The model under review builds one solid part; all positions refer to its coordinate system, in mm. A direction names the side the tool comes from. Give positions to 0.01 mm unless a question says otherwise; leave off trailing zeros. Loops run counter-clockwise (first coordinate to the right, second up) from the corner with the lowest first, then second, coordinate; pieces in that order, holes last. Notation, with made-up numbers: M 67,-4 L 73,-4 A18 cw 73,23 Z; hole C -19,18.25 d1. An arc over 180 degrees is marked long. One line per item, written item: value. Start each with the question number.
Q1. We need section B-B on y = -50.5. Write out the cut boundary in (x, z).
Q2. For pin 1 (3 mm diameter, centred on x = -85.68, y = -111.2, fed in from -Z); pin 2 (3 mm diameter, centred on x = 0, y = -188.04, fed in from +Z); pin 3 (1.5 mm diameter, centred on x = -11, z = 1.5, fed in from -Y); pin 4 (1.5 mm diameter, centred on x = -14, z = 2, fed in from +Y), all flat-tipped, find the tip position at first contact; note any pin that passes through.
Q3. For faces 4 (the face through (-32.17, -58.77, -1.48)), 5 (the face through (1.15, -190.26, 1.52)), list the 3-axis set-ups (+Z, -Z, +X, -X, +Y, -Y) from which the entire face can be reached by the end or side of a thin tool; tool diameter is ignored.
Q4. We need section D-D on y = -158.5. Write out the cut boundary in (x, z).
Q5. We need section C-C on x = -142. Write out the cut boundary in (y, z), plus the area to 3 significant figures.
Q6. We need section A-A on z = -1.2. Write out the cut boundary in (x, y), plus the area to 3 significant figures.
Q7. To check wall thickness, follow line 1 along Y through (x, z) = (0, 2.1); line 2 along X through (y, z) = (-120, 0.2); line 3 along X through (y, z) = (-118, 0.4). State the ranges of each line that lie inside material, in increasing order. Write a range as from..to.
Q8. Mouldability with a two-part tool opening along Y and no side actions: class faces 1 (the face through (-34, -57, -3)), 2 (the face through (-84.53, -149.05, 1.48)), 3 (the face through (-97.158, -125.157, 1.521)) as released by +Y, released by -Y, zero draft, split by the parting line, or undercut.
Autodesk Inventor part; units mm, degrees
ref_plane "YZ Plane" through (0, 0, 0) normal (1, 0, 0) x (0, 1, 0)
ref_plane "XZ Plane" through (0, 0, 0) normal (0, 1, 0) x (-1, 0, 0)
ref_plane "XY Plane" through (0, 0, 0) normal (0, 0, 1) x (1, 0, 0)
sketch "Sketch1" plane through (0, 0, 0) normal (0, 0, 1) x (1, 0, 0)
  line L0 (-169.4076, 105.3841) -> (50.098, -274.8108)
  circle A0 centre (-54.282, -94.0192) radius 2.75
  circle A1 centre (0, 0) radius 8.5
  circle A2 centre (-162.8461, -94.0192) radius 8.5
  circle A3 centre (0, -188.0385) radius 8.5
  line L1 (0, 0) -> (0, -188.0385)
  line L2 (0, -188.0385) -> (-162.8461, -94.0192)
  line L3 (-162.8461, -94.0192) -> (0, 0)
  line L4 (38.7758, 32.2022) -> (-208.87, -110.7762)
  line L5 (8.5, -269.7975) -> (8.5, 26.6982)
  line L6 (49.2969, -226.315) -> (-222.0406, -69.6582)
  circle A4 centre (-54.282, -94.0192) radius 2.75
  point P0 (8.5, -188.0385)
  point P1 (8.5, 0)
  point P2 (-4.25, 7.3612)
  point P3 (-167.0961, -86.658)
  point P4 (-167.0961, -101.3805)
  point P5 (-4.25, -195.3997)
  dimension "d0" = 17
  dimension "d3" = 360
  dimension "d49" = 5.5
extrude "Extrusion1" add sketch "Sketch1" along normal blind 3 contours L4 A1 L3 L0 | L0 L3 A2 L4 | L3 A1 L1 A3 L0 A0 | L0 A0 A3 L2 A2 L3 | A1 L1 L3 | A2 L3 L2 | A2 L2 L3 | L3 L1 A1 | L5 A3 L1 A1 | A2 L2 A3 L6 | A3 L0 L1 | A3 L2 L0 | A3 L1 L0 | L0 L2 A3
sketch "Sketch2" plane through (0, 0, 3) normal (0, 0, 1) x (1, 0, 0)
  circle A0 centre (0, 0) radius 2.5
  line L0 (-169.4076, 105.3841) -> (50.098, -274.8108)
  line L1 (-169.4076, -293.4225) -> (50.098, 86.7723)
  circle A1 centre (-54.282, -94.0192) radius 2.75
  circle A2 centre (-162.8461, -94.0192) radius 2.5
  circle A3 centre (0, -188.0385) radius 2.5
  point P0 (-54.282, -94.0192)
  dimension "d7" = 5
  dimension "d10" = 360
extrude "Extrusion2" cut sketch "Sketch2" against normal up to surface (3 mm away) contours A0 L1 | A3 L0 | L0 A3 | L1 A0 | A2
sketch "Sketch3" plane through (0, 0, 0) normal (0, 0, -1) x (-1, 0, 0)
  circle A0 centre (54.282, -94.0192) radius 2.75
  circle A1 centre (0, 0) radius 2.5
  line L0 (0, 0) -> (54.282, -94.0192)
  circle A2 centre (162.8461, -94.0192) radius 2.5
  line L1 (54.282, -94.0192) -> (162.8461, -94.0192)
  circle A3 centre (0, -188.0385) radius 2.5
  line L2 (54.282, -94.0192) -> (0, -188.0385)
  line L3 (0, 0) -> (32.5, -56.2917)
  circle A4 centre (32.5, -56.2917) radius 1.5
  circle A5 centre (32.5, -56.2917) radius 2.5
  circle A6 centre (32.5, -131.7468) radius 2.5
  circle A7 centre (32.5, -131.7468) radius 1.5
  circle A8 centre (97.8461, -94.0192) radius 2.5
  circle A9 centre (97.8461, -94.0192) radius 1.5
  dimension "d14" = 65
  dimension "d15" = 3
  dimension "d16" = 5
  dimension "d19" = 360
extrude "Extrusion3" add sketch "Sketch3" along normal blind 3 contours A6 L2 A7 | L2 A7 A6 | A5 L0 A4 | L0 A4 A5 | A8 L1 A9 | L1 A9 A8
sketch "Sketch4" plane through (0, 0, 0) normal (0, 0, -1) x (-1, 0, 0)
  circle A0 centre (32.5, -56.2917) radius 1.5
  circle A1 centre (32.5, -131.7468) radius 1.5
  circle A2 centre (97.8461, -94.0192) radius 1.5
  point P0 (0, 0)
extrude "Extrusion4" cut sketch "Sketch4" against normal blind 3
sketch "Sketch5" plane through (0, 0, 3) normal (0, 0, 1) x (1, 0, 0)
  circle A0 centre (-32.5, -56.2917) radius 1.5
  circle A1 centre (-32.5, -131.7468) radius 1.5
  line L0 (-32.5, -56.2917) -> (2.5, -56.2917)
  line L1 (2.5, -56.2917) -> (2.5, -131.7468)
  line L2 (2.5, -131.7468) -> (-32.5, -131.7468)
  line L3 (-32.5, -131.7468) -> (-32.5, -56.2917)
  circle A2 centre (2.5, -56.2917) radius 1.5
  circle A3 centre (2.5, -131.7468) radius 1.5
  point P0 (0, 0)
  dimension "d25" = 35
  dimension "d26" = 3
  dimension "d27" = 3
extrude "Extrusion5" cut sketch "Sketch5" against normal blind 3 contours A2 L1 L0 | L0 L1 A2 | A3 L2 L1 | L1 L2 A3
sketch "Sketch7" plane through (0, 0, 3) normal (0, 0, 1) x (1, 0, 0)
  circle A0 centre (-32.5, -56.2917) radius 1.5
  circle A1 centre (2.5, -131.7468) radius 1.5
  line L0 (-32.5, -56.2917) -> (2.5, -131.7468)
  circle A2 centre (2.5, -56.2917) radius 1.5
  circle A3 centre (-32.5, -131.7468) radius 1.5
  line L1 (2.5, -56.2917) -> (-32.5, -131.7468)
  line L2 (2.5, -60.5192) -> (-32.5, -60.5192)
  line L3 (-32.5, -60.5192) -> (-32.5, -127.5192)
  line L4 (-32.5, -127.5192) -> (2.5, -127.5192)
  line L5 (2.5, -127.5192) -> (2.5, -60.5192)
  line L6 (2.5, -60.5192) -> (-32.5, -127.5192) construction
  line L7 (-32.5, -60.5192) -> (2.5, -127.5192) construction
  point P0 (0, 0)
  point P1 (-15, -94.0192)
  dimension "d36" = 35
  dimension "d37" = 67
extrude "Extrusion7" cut sketch "Sketch7" against normal blind 3 contours L2 L1 L0 | L0 L1 L4 L3 L2 | L1 L2 L5 L4 L0 | L0 L4 L1
sketch "Sketch8" plane through (0, 0, 3) normal (0, 0, 1) x (1, 0, 0)
  line L0 (-53.465, -129.8041) -> (-67.565, -154.226)
  line L1 (-67.565, -154.226) -> (-99.7811, -135.626)
  line L2 (-99.7811, -135.626) -> (-85.6811, -111.2041)
  line L3 (-85.6811, -111.2041) -> (-53.465, -129.8041)
  circle A0 centre (-67.565, -154.226) radius 1.25
  circle A1 centre (-53.465, -129.8041) radius 1.25
  circle A2 centre (-99.7811, -135.626) radius 1.25
  circle A3 centre (-85.6811, -111.2041) radius 1.25
  line L4 (-167.0961, -101.3805) -> (-4.25, -195.3997)
  line L5 (-167.0961, -101.3805) -> (-4.25, -195.3997)
  line L6 (-85.673, -148.3901) -> (-48.0406, -83.2087)
  circle A4 centre (-54.282, -94.0192) radius 2.75
  point P0 (0, 0)
  point P1 (-69.573, -120.5041)
  dimension "d40" = 28.2
  dimension "d41" = 37.2
  dimension "d42" = 2.5
  dimension "d43" = 2.5
  dimension "d44" = 2.5
  dimension "d45" = 2.5
  dimension "d46" = 4
extrude "Extrusion8" cut sketch "Sketch8" against normal blind 10 contours L3 A1 L0 | L0 A1 L3 | A0 L1 L0 | L0 L1 A0 | A3 L2 L3 | L3 L2 A3 | A2 L2 L1 | L1 L2 A2
sketch "Sketch9" plane through (0, 0, 3) normal (0, 0, 1) x (1, 0, 0)
  circle A0 centre (-54.282, -46.3878) radius 7.5
  circle A1 centre (-95.532, -70.2035) radius 7.5
  circle A2 centre (-54.282, -141.6506) radius 7.5
  circle A3 centre (-95.532, -117.8349) radius 7.5
  point P0 (0, 0)
extrude "Extrusion9" cut sketch "Sketch9" against normal up to surface (3 mm away)
sketch "Sketch10" plane through (0, 0, 3) normal (0, 0, 1) x (1, 0, 0)
  line L0 (-140.8461, -109.2592) -> (-140.8461, -78.7792)
  line L1 (-140.8461, -78.7792) -> (-123.0661, -78.7792)
  circle A0 centre (-131.9561, -81.3192) radius 1.27
  circle A1 centre (-131.9561, -106.7192) radius 1.27
  point P0 (0, 0)
extrude "Extrusion10" cut sketch "Sketch10" against normal blind 10
properties part number "second_etage" material "PET Plastic"
Solved:
1. outline: M -104.47,0 L -60.55,0 L -60.55,3 L -104.47,3 Z; M -48.01,0 L 8.5,0 L 8.5,3 L -48.01,3 Z
2. pin 1: z = 0
2. pin 2: through
2. pin 3: y = -191.94
2. pin 4: y = 2.17
3. face 4: -Z
3. face 5: +Z, -Z
4. outline: M -68.16,0 L 8.5,0 L 8.5,3 L -68.16,3 Z
5. outline: M -115.87,0 L -72.17,0 L -72.17,3 L -115.87,3 Z
5. area: 131 mm2
6. outline: C -97.85,-94.02 d5; C -32.5,-131.75 d5; C -32.5,-56.29 d5; hole C -97.85,-94.02 d3; hole C -32.5,-131.75 d3; hole C -32.5,-56.29 d3
6. area: 37.7 mm2
7. line 1: -196.54..-190.54, -185.54..-127.52, -60.52..-2.5, 2.5..8.5
7. line 2: -134.85..-102.71, -88.35..-32.5, 2.5..8.5
7. line 3: -138.31..-103.03, -88.03..-32.5, 2.5..8.5
8. face 1: zero draft
8. face 2: released by -Y
8. face 3: undercut
